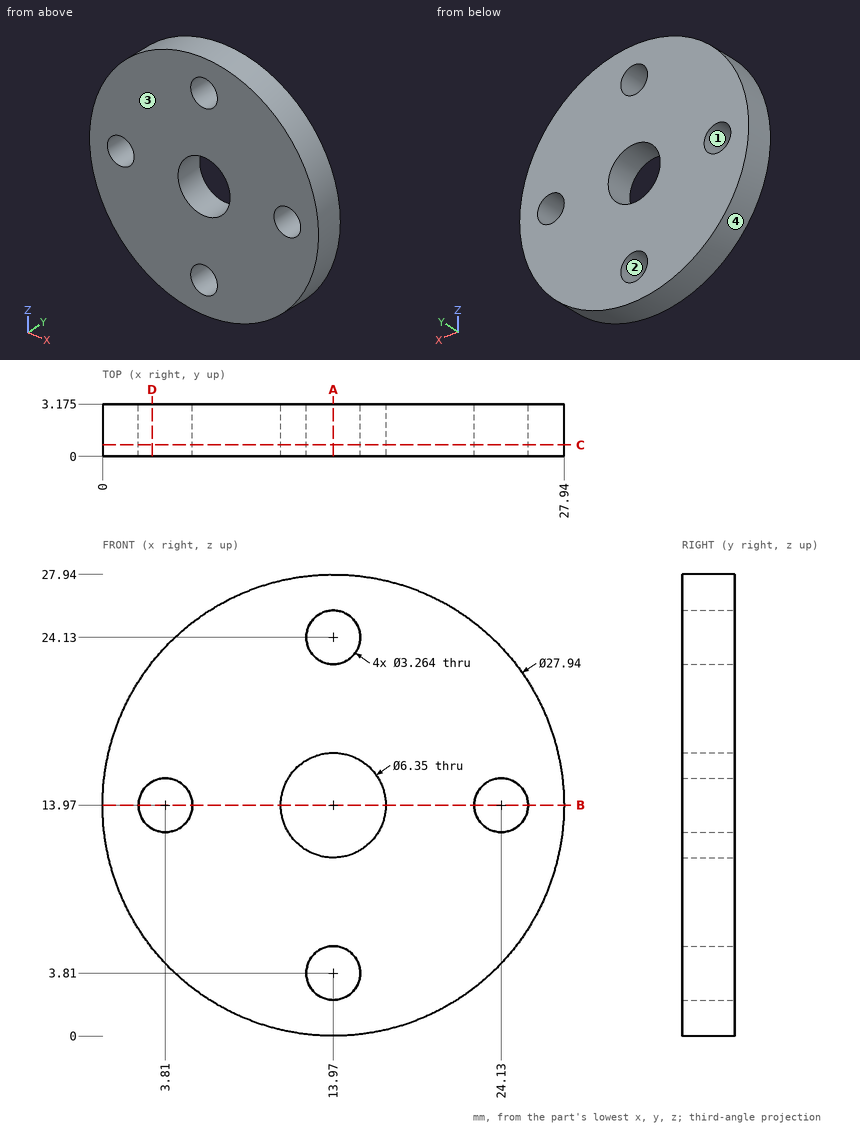
Print and shaded views of the part. All mm, measured from the part's lowest x, y and z. Coordinates: 2 decimals unless noted, no trailing zeros. Order: outer loops, then holes, each group sorted by start corner. A loop starts at its lowest first (then second) coordinate and runs counter-clockwise, first axis right, second up. Notation, with made-up numbers: (-21, 8) - (22, 8) arc R29 ccw to (22, 29) - close; hole circle Ø1 at (56, 56.25). An arc over 180 degrees is marked (long way). Return JSON: item names as keys, results as strings. Group by question number.
Item 1: Cut at C-C (y = 0.7). List the corners of the cut face in (x, z) (3 decimals).
Item 2: Pull direction Z, two halves, no side cores. Call the marked faces 1, 2, 3 and 4: pulls with the +Z half, pulls with the -Z half, needs draft (parallel to the pull), parting line crosses it, or undercut.
Item 3: Cut at B-B (z = 13.97). List the corners of the cut face in (x, y) (3 decimals), plus the area to 3 significant figures.
Item 4: Cut at A-A (x = 13.97). List the corners of the cut face in (y, z) (3 decimals), plus the area to 3 significant figures.
Item 5: Cut at D-D (x = 3). List the corners of the cut face in (y, z) (3 decimals).
Item 6: Pin check, flat tips, straight feed: pin 1 (1 mm diameter, centred on y = 2, z = 11.5, fed in from -X); pin 2 (1 mm diameter, centred on y = 1, z = 20, fed in from -X); pin 3 (2.5 mm diameter, centred on x = 13.97, z = 24.13, fed in from +Y). Stop position of each tip, or through.
Item 7: Drill centre lines: probe 1 along Z at (x, y) = (13.97, 0.8) (3 decimals); probe 2 along Z at (x, y) = (13.5, 2.45); probe 3 along X at (y, z) = (2.8, 25). Where is each one in solid material? Low to high. Write a range as from..to.
Check values:
{
 "1": {"outline": "circle Ø27.94 at (13.97, 13.97); hole circle Ø3.264 at (3.81, 13.97); hole circle Ø6.35 at (13.97, 13.97); hole circle Ø3.264 at (13.97, 3.81); hole circle Ø3.264 at (13.97, 24.13); hole circle Ø3.264 at (24.13, 13.97)"},
 "2": {"face 1": "undercut", "face 2": "undercut", "face 3": "needs draft", "face 4": "parting line crosses it"},
 "3": {"outline": "(0, 0) - (2.178, 0) - (2.178, 3.175) - (0, 3.175) - close; (5.442, 0) - (10.795, 0) - (10.795, 3.175) - (5.442, 3.175) - close; (17.145, 0) - (22.498, 0) - (22.498, 3.175) - (17.145, 3.175) - close; (25.762, 0) - (27.94, 0) - (27.94, 3.175) - (25.762, 3.175) - close", "area": "47.8 mm2"},
 "4": {"outline": "(0, 0) - (3.175, 0) - (3.175, 2.178) - (0, 2.178) - close; (0, 5.442) - (3.175, 5.442) - (3.175, 10.795) - (0, 10.795) - close; (0, 17.145) - (3.175, 17.145) - (3.175, 22.498) - (0, 22.498) - close; (0, 25.762) - (3.175, 25.762) - (3.175, 27.94) - (0, 27.94) - close", "area": "47.8 mm2"},
 "5": {"outline": "(0, 5.32) - (3.175, 5.32) - (3.175, 12.553) - (0, 12.553) - close; (0, 15.387) - (3.175, 15.387) - (3.175, 22.62) - (0, 22.62) - close"},
 "6": {"pin 1": "stops at x = 0.14", "pin 2": "stops at x = 1.14", "pin 3": "passes through"},
 "7": {"probe 1": "z = 0..2.178, 5.442..10.795, 17.145..22.498, 25.762..27.94", "probe 2": "z = 0.01..2.25, 5.37..10.83, 17.11..22.57, 25.69..27.93", "probe 3": "x = 5.4..12.59, 15.35..22.54"}
}
